```python
from build123d import *

# Parameters (mm, degrees)
F0_R     = 69.85
F1_DEPTH = 4.7625
F3_DEPTH = 25.4


with BuildPart() as f1:
    # F0 (on Top) → F1 (new body)
    with BuildSketch(Plane.XY):
        Circle(F0_R)
    extrude(amount=F1_DEPTH)

    # F2 (on face) → F3 (cut)
    with BuildSketch(Plane.XY.offset(4.7625)):
        with BuildLine():
            ThreePointArc((12.12932521, 68.7888215479), (6.0878286309, 69.5841996617), (0, 69.85))
            Line((0, 69.85), (0, 63.5))
            ThreePointArc((0, 63.5), (5.5343896645, 63.2583633288), (11.0266592819, 62.5352923163))
            Line((11.0266592819, 62.5352923163), (12.12932521, 68.7888215479))
        make_face()
        with BuildLine():
            ThreePointArc((-12.12932521, 68.7888215479), (-18.0785103004, 67.4699189663), (-23.8901070113, 65.6375295619))
            Line((-23.8901070113, 65.6375295619), (-21.7182791012, 59.6704814199))
            ThreePointArc((-21.7182791012, 59.6704814199), (-16.435009364, 61.3362899694), (-11.0266592819, 62.5352923163))
            Line((-11.0266592819, 62.5352923163), (-12.12932521, 68.7888215479))
        make_face()
        with BuildLine():
            ThreePointArc((-34.925, 60.4918744543), (-40.0643140791, 57.2177702936), (-44.8987145366, 53.5082043519))
            Line((-44.8987145366, 53.5082043519), (-40.8170132151, 48.6438221381))
            ThreePointArc((-40.8170132151, 48.6438221381), (-36.4221037083, 52.0161548124), (-31.75, 54.9926131403))
            Line((-31.75, 54.9926131403), (-34.925, 60.4918744543))
        make_face()
        with BuildLine():
            ThreePointArc((-53.5082043519, 44.8987145366), (-57.2177702936, 40.0643140791), (-60.4918744543, 34.925))
            Line((-60.4918744543, 34.925), (-54.9926131403, 31.75))
            ThreePointArc((-54.9926131403, 31.75), (-52.0161548124, 36.4221037083), (-48.6438221381, 40.8170132151))
            Line((-48.6438221381, 40.8170132151), (-53.5082043519, 44.8987145366))
        make_face()
        with BuildLine():
            ThreePointArc((-65.6375295619, 23.8901070113), (-67.4699189663, 18.0785103004), (-68.7888215479, 12.12932521))
            Line((-68.7888215479, 12.12932521), (-62.5352923163, 11.0266592819))
            ThreePointArc((-62.5352923163, 11.0266592819), (-61.3362899694, 16.435009364), (-59.6704814199, 21.7182791012))
            Line((-59.6704814199, 21.7182791012), (-65.6375295619, 23.8901070113))
        make_face()
        with BuildLine():
            ThreePointArc((-69.85, 0), (-69.5841996617, -6.0878286309), (-68.7888215479, -12.12932521))
            Line((-68.7888215479, -12.12932521), (-62.5352923163, -11.0266592819))
            ThreePointArc((-62.5352923163, -11.0266592819), (-63.2583633288, -5.5343896645), (-63.5, 0))
            Line((-63.5, 0), (-69.85, 0))
        make_face()
        with BuildLine():
            ThreePointArc((-65.6375295619, -23.8901070113), (-63.3055989245, -29.5198855826), (-60.4918744543, -34.925))
            Line((-60.4918744543, -34.925), (-54.9926131403, -31.75))
            ThreePointArc((-54.9926131403, -31.75), (-57.5505444768, -26.8362596205), (-59.6704814199, -21.7182791012))
            Line((-59.6704814199, -21.7182791012), (-65.6375295619, -23.8901070113))
        make_face()
        with BuildLine():
            ThreePointArc((-53.5082043519, -44.8987145366), (-49.3914086659, -49.3914086659), (-44.8987145366, -53.5082043519))
            Line((-44.8987145366, -53.5082043519), (-40.8170132151, -48.6438221381))
            ThreePointArc((-40.8170132151, -48.6438221381), (-44.9012806053, -44.9012806053), (-48.6438221381, -40.8170132151))
            Line((-48.6438221381, -40.8170132151), (-53.5082043519, -44.8987145366))
        make_face()
        with BuildLine():
            ThreePointArc((-34.925, -60.4918744543), (-29.5198855826, -63.3055989245), (-23.8901070113, -65.6375295619))
            Line((-23.8901070113, -65.6375295619), (-21.7182791012, -59.6704814199))
            ThreePointArc((-21.7182791012, -59.6704814199), (-26.8362596205, -57.5505444768), (-31.75, -54.9926131403))
            Line((-31.75, -54.9926131403), (-34.925, -60.4918744543))
        make_face()
        with BuildLine():
            ThreePointArc((-12.12932521, -68.7888215479), (-6.0878286309, -69.5841996617), (0, -69.85))
            Line((0, -69.85), (0, -63.5))
            ThreePointArc((0, -63.5), (-5.5343896645, -63.2583633288), (-11.0266592819, -62.5352923163))
            Line((-11.0266592819, -62.5352923163), (-12.12932521, -68.7888215479))
        make_face()
        with BuildLine():
            ThreePointArc((12.12932521, -68.7888215479), (18.0785103004, -67.4699189663), (23.8901070113, -65.6375295619))
            Line((23.8901070113, -65.6375295619), (21.7182791012, -59.6704814199))
            ThreePointArc((21.7182791012, -59.6704814199), (16.435009364, -61.3362899694), (11.0266592819, -62.5352923163))
            Line((11.0266592819, -62.5352923163), (12.12932521, -68.7888215479))
        make_face()
        with BuildLine():
            ThreePointArc((34.925, -60.4918744543), (40.0643140791, -57.2177702936), (44.8987145366, -53.5082043519))
            Line((44.8987145366, -53.5082043519), (40.8170132151, -48.6438221381))
            ThreePointArc((40.8170132151, -48.6438221381), (36.4221037083, -52.0161548124), (31.75, -54.9926131403))
            Line((31.75, -54.9926131403), (34.925, -60.4918744543))
        make_face()
        with BuildLine():
            ThreePointArc((53.5082043519, -44.8987145366), (57.2177702936, -40.0643140791), (60.4918744543, -34.925))
            Line((60.4918744543, -34.925), (54.9926131403, -31.75))
            ThreePointArc((54.9926131403, -31.75), (52.0161548124, -36.4221037083), (48.6438221381, -40.8170132151))
            Line((48.6438221381, -40.8170132151), (53.5082043519, -44.8987145366))
        make_face()
        with BuildLine():
            ThreePointArc((65.6375295619, -23.8901070113), (67.4699189663, -18.0785103004), (68.7888215479, -12.12932521))
            Line((68.7888215479, -12.12932521), (62.5352923163, -11.0266592819))
            ThreePointArc((62.5352923163, -11.0266592819), (61.3362899694, -16.435009364), (59.6704814199, -21.7182791012))
            Line((59.6704814199, -21.7182791012), (65.6375295619, -23.8901070113))
        make_face()
        with BuildLine():
            ThreePointArc((69.85, 0), (69.5841996617, 6.0878286309), (68.7888215479, 12.12932521))
            Line((68.7888215479, 12.12932521), (62.5352923163, 11.0266592819))
            ThreePointArc((62.5352923163, 11.0266592819), (63.2583633288, 5.5343896645), (63.5, 0))
            Line((63.5, 0), (69.85, 0))
        make_face()
        with BuildLine():
            ThreePointArc((65.6375295619, 23.8901070113), (63.3055989245, 29.5198855826), (60.4918744543, 34.925))
            Line((60.4918744543, 34.925), (54.9926131403, 31.75))
            ThreePointArc((54.9926131403, 31.75), (57.5505444768, 26.8362596205), (59.6704814199, 21.7182791012))
            Line((59.6704814199, 21.7182791012), (65.6375295619, 23.8901070113))
        make_face()
        with BuildLine():
            ThreePointArc((53.5082043519, 44.8987145366), (49.3914086659, 49.3914086659), (44.8987145366, 53.5082043519))
            Line((44.8987145366, 53.5082043519), (40.8170132151, 48.6438221381))
            ThreePointArc((40.8170132151, 48.6438221381), (44.9012806053, 44.9012806053), (48.6438221381, 40.8170132151))
            Line((48.6438221381, 40.8170132151), (53.5082043519, 44.8987145366))
        make_face()
        with BuildLine():
            ThreePointArc((34.925, 60.4918744543), (29.5198855826, 63.3055989245), (23.8901070113, 65.6375295619))
            Line((23.8901070113, 65.6375295619), (21.7182791012, 59.6704814199))
            ThreePointArc((21.7182791012, 59.6704814199), (26.8362596205, 57.5505444768), (31.75, 54.9926131403))
            Line((31.75, 54.9926131403), (34.925, 60.4918744543))
        make_face()
    extrude(amount=-F3_DEPTH, mode=Mode.SUBTRACT)


solid = f1.part
```
Input: part model. Units: mm. Frame: model coordinates. A direction names the side the tool comes from. Give positions to 0.01 mm unless a question says otherwise; leave off trailing zeros. Loops run counter-clockwise (first coordinate to the right, second up) from the corner with the lowest first, then second, coordinate; pieces in that order, holes last.
1) Section query C-C on x = 43. Return the cut outline in (y, z), and give its area (3 significant figures).
A:
outline: (-51.25, 0) - (46.73, 0) - (46.73, 4.76) - (-51.25, 4.76) - close; (51.25, 0) - (55.05, 0) - (55.05, 4.76) - (51.25, 4.76) - close
area: 485 mm2
2) Section query A-A on x = -51.5. Return the cut outline in (y, z), and give its area (3 significant figures).
A:
outline: (-43.21, 0) - (37.15, 0) - (37.15, 4.76) - (-43.21, 4.76) - close; (43.21, 0) - (47.19, 0) - (47.19, 4.76) - (43.21, 4.76) - close
area: 402 mm2
3) Contact query for flat-ended pins moving along their axis: pin 1 (2.5 mm diameter, centred on y = -65.5, z = 2, fed in from -X); pin 2 (1.5 mm diameter, centred on x = 2, z = 3, fed in from +Y); pin 3 (1.5 mm diameter, centred on x = 47.5, z = 4, fed in from -Y). Output: stop coordinate, or through.
A:
pin 1: stops at x = -23.89
pin 2: stops at y = 63.49
pin 3: stops at y = -51.9
4) Line query: L1, parallel to X at y = -55.5, z = 0.3; L2, parallel to Y at x = 57, z = 4.4; L3, parallel to X at y = 55.5, z = 1.2. Output: solid intervals per line, ascending.
A:
L1: x = -42.41 to -32.04, -30.85 to 32.04
L2: y = -32.91 to 27.99, 32.91 to 40.37
L3: x = -32.04 to 30.85, 32.04 to 42.41
5) Reachability of faces 1 (the flat face through (-11.57, -65.62, 2.41)), 2 (the flat face through (51.04, -42.83, 2.41)), 3 (the flat face through (-57.78, 33.36, 2.41)), 4 (the flat face through (-67, 0, 2)), 5 (the flat face through (65.706, -11.586, 2.415)) from +Z, -Z, +X, -X, +Y, -Y: full face, straight path, thin tool, end or side. Return the list, or none.
A:
face 1: +Z, -Z, -Y
face 2: +Z, -Z, +X
face 3: +Z, -Z, +Y
face 4: +Z, -Z, -X
face 5: +Z, -Z
6) Section query D-D on y = 28. Return the cut outline in (x, z).
A:
outline: (-63.99, 0) - (56.99, 0) - (56.99, 4.76) - (-63.99, 4.76) - close
7) Section query B-B on y = -9. Return the cut outline in (x, z).
A:
outline: (-62.86, 0) - (69.27, 0) - (69.27, 4.76) - (-62.86, 4.76) - close
